from build123d import *

# Parameters (mm, degrees)
BOSS_EXTRU_1_DEPTH       = 9.5
ESQUISSE3_R              = 2.5
ENL_V_MAT_EXTRU_40_DEPTH = 10
BOSS_EXTRU_2_DEPTH       = 2
CONG_1_R                 = 2
ESQUISSE5_R              = 6.5
BOSS_EXTRU_3_DEPTH       = 1.5
CONG_2_R                 = 0.75
ESQUISSE6_R              = 5.5
BOSS_EXTRU_4_DEPTH       = 0.5
ESQUISSE7_R              = 3
BOSS_EXTRU_5_DEPTH       = 3.5


with BuildPart() as part:
    # Esquisse1 → Boss.-Extru.1 (new, symmetric)
    with BuildSketch(Plane(origin=(0, 0, 0), x_dir=(0, 0, -1), z_dir=(1, 0, 0))):
        Polygon((0, 0), (4, 0), (4, -7), (6, -7), (6, 0), (33, 0), (33, 40), (6, 40), (6, 47), (4, 47), (4, 40), (0, 40), align=None)
    extrude(amount=BOSS_EXTRU_1_DEPTH, both=True)

    # Esquisse3 → Enlèv. mat.-Extru.40 (cut)
    with BuildSketch(Plane.XY.offset(-4)):
        with Locations((5, 44.4)):
            Circle(ESQUISSE3_R)
        with Locations((-5, 44.4)):
            Circle(ESQUISSE3_R)
        with Locations((5, -4.4)):
            Circle(ESQUISSE3_R)
        with Locations((-5, -4.4)):
            Circle(ESQUISSE3_R)
    extrude(amount=-ENL_V_MAT_EXTRU_40_DEPTH, mode=Mode.SUBTRACT)

    # Esquisse4 → Boss.-Extru.2 (add)
    with BuildSketch(Plane.XY):
        with BuildLine():
            Line((-9.034932354, 5), (9.018945802, 5))
            Line((9.018945802, 5), (9.018945802, 29.110938176))
            ThreePointArc((9.018945802, 29.110938176), (-0.007993276, 40), (-9.034932354, 29.110938176))
            Line((-9.034932354, 29.110938176), (-9.034932354, 5))
        make_face()
    extrude(amount=BOSS_EXTRU_2_DEPTH)

    # Congé1
    cong_1_edges = [part.edges().sort_by_distance(p)[0] for p in [
        (-9.5, 20, -33),
        (0, 40, -33),
        (0, 0, -33),
        (9.5, 20, -33),
    ]]
    fillet(cong_1_edges, radius=CONG_1_R)

    # Esquisse5 → Boss.-Extru.3 (add)
    with BuildSketch(Plane.XY.offset(2)):
        with Locations(Location((0, 31.4090745, 0), (0, 0, 180))):
            Circle(ESQUISSE5_R)
    extrude(amount=BOSS_EXTRU_3_DEPTH)

    # Congé2
    cong_2_edges = [part.edges().sort_by_distance(p)[0] for p in [
        (6.5, 31.4090745, 3.5),
    ]]
    fillet(cong_2_edges, radius=CONG_2_R)

    # Esquisse6 → Boss.-Extru.4 (add)
    with BuildSketch(Plane.XY.offset(3.5)):
        with Locations((0, 31.4090745)):
            Circle(ESQUISSE6_R)
    extrude(amount=BOSS_EXTRU_4_DEPTH)

    # Esquisse7 → Boss.-Extru.5 (add)
    with BuildSketch(Plane.XY.offset(4)):
        with Locations((0, 31.4090745)):
            Circle(ESQUISSE7_R)
    extrude(amount=BOSS_EXTRU_5_DEPTH)


solid = part.part
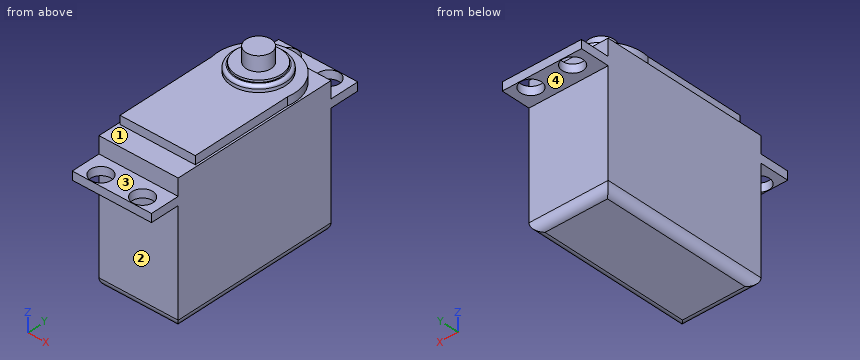
The listing builds one solid part. Answer for the finished solid, in the listing's coordinates (mm). Face numbers are marked on the shaded views. A direction names the side the tool comes from. Round coordinates to 2 decimals unless told otherwise and drop trailing zeros. Write each loop counter-clockwise with the first axis right and the second up, starting at its lowest first coordinate (ties: lowest second). Pieces come first, ordered by that corner, then holes. Notation, with made-up numbers: M -30,7.5 L -12,7.5 A12 ccw -12,11.5 Z; hole C 82.5,86.25 d7. An arc over 180 degrees is marked long. Write each question's results on one line, items separated by ' | '. Start each with the question number.
(1) Each of these flat-tipped pins is pushed along its axis until it touches: P1, Ø3.5, axis at x = 1, y = -4.5, coming from the +Z side; P2, Ø5, axis at x = 6, z = -14.5, coming from the +Y side; P3, Ø1.2, axis at x = -4, z = -2.5, coming from the -Y side; P4, Ø3, axis at x = -5, y = -4.4, coming from the +Z side. Where does it stop, or does it pass through?
(2) Find the intervals of material crossed by line 1 (Y direction, x = 7.5, z = -24); line 2 (Z direction, x = 7.75, y = 40.5); line 3 (Z direction, x = 6, y = 7), in increasing order.
(3) The part is cut by section A-A, the plane y = 44.4. Write down the section's boundary in (x, z).
(4) For the marked faces 1, 2, 3 and 4, determine the directions among +Z, -Z, +X, -X, +Y, -Y from which every point of the face is accessible in a straight line to the end or side of a thin tool.
(5) The part is cut by section C-C, the plane x = 4.5. Give the number of separate pieces and of enclosed holes in the cut face, and give its area (3 significant figures).
(6) The part is cut by section B-B, the plane y = 9. Write down the section's boundary in (x, z), and give its area (3 significant figures).
(7) The part is cut by section D-D, the plane z = -1. Write down the section's boundary in (x, y).
Worked answers:
1) P1: stops at z = -4 | P2: stops at y = 40 | P3: stops at y = 0 | P4: passes through
2) line 1: y = 0 to 40 | line 2: z = -6 to -4 | line 3: z = -33 to 2
3) outline: M -9.5,-6 L -7.5,-6 L -7.5,-4 L -9.5,-4 Z; M -2.5,-6 L 2.5,-6 L 2.5,-4 L -2.5,-4 Z; M 7.5,-6 L 9.5,-6 L 9.5,-4 L 7.5,-4 Z
4) face 1: +Z | face 2: -Z, +X, -X, -Y | face 3: +Z, +X, -X, -Y | face 4: -Z, +X, -X, +Y
5) separate pieces: 3 | enclosed holes: 0 | area: 1,410 mm²
6) outline: M -9.5,-31 A2 ccw -7.5,-33 L 7.5,-33 A2 ccw 9.5,-31 L 9.5,0 L 9.02,0 L 9.02,2 L -9.03,2 L -9.03,0 L -9.5,0 Z | area: 661 mm²
7) outline: M -9.5,0 L 9.5,0 L 9.5,40 L -9.5,40 Z
